```python
from build123d import *

# Parameters (mm, degrees)
SKETCH2_W           = 40
SKETCH2_H           = 20
SKETCH2_R           = 1.5
BOSS_EXTRUDE1_DEPTH = 3
BOSS_EXTRUDE2_DEPTH = 20
SKETCH4_R           = 1.5
CUT_EXTRUDE1_DEPTH  = 20
FILLET2_R           = 2.5


with BuildPart() as part:
    # Sketch2 → Boss-Extrude1 (new body)
    with BuildSketch(Plane(origin=(0, 0, 0), x_dir=(1, 0, 0), z_dir=(0, 1, 0))):
        with Locations((20, 10)):
            Rectangle(SKETCH2_W, SKETCH2_H)
        with Locations(Location((5, 5, 0), (0, 0, 270))):
            Circle(SKETCH2_R, mode=Mode.SUBTRACT)
        with Locations(Location((15, 5, 0), (0, 0, 270))):
            Circle(SKETCH2_R, mode=Mode.SUBTRACT)
        with Locations(Location((15, 15, 0), (0, 0, 270))):
            Circle(SKETCH2_R, mode=Mode.SUBTRACT)
        with Locations(Location((5, 15, 0), (0, 0, 270))):
            Circle(SKETCH2_R, mode=Mode.SUBTRACT)
    extrude(amount=BOSS_EXTRUDE1_DEPTH)

    # Sketch3 → Boss-Extrude2 (add)
    with BuildSketch(Plane(origin=(0, 3, 0), x_dir=(1, 0, 0), z_dir=(0, 1, 0))):
        Polygon((22.097168491, 18), (35.975848148, 4.121320344), (33.854527804, 2), (19.975848148, 15.878679656), align=None)
        Polygon((35.878679656, 8.461129522), (28.461129522, 15.878679656), (30.582449865, 18), (38, 10.582449865), align=None)
    extrude(amount=BOSS_EXTRUDE2_DEPTH)

    # Sketch4 → Cut-Extrude1 (cut)
    with BuildSketch(Plane(origin=(24.291224933, 0, -24.291224933), x_dir=(-0.7071067811865372, 0, -0.7071067811865579), z_dir=(0.7071067811865579, 0, -0.7071067811865372))):
        with Locations((-13.897135624, 18)):
            Circle(SKETCH4_R)
        with Locations((-13.897135624, 13)):
            Circle(SKETCH4_R)
        with Locations((-13.897135624, 8)):
            Circle(SKETCH4_R)
    extrude(amount=-CUT_EXTRUDE1_DEPTH, mode=Mode.SUBTRACT)

    # Fillet2
    fillet2_edges = [part.edges().sort_by_distance(p)[0] for p in [
        (34.915187976, 3, -3.060660172),
        (34.915187976, 23, -3.060660172),
        (36.939339828, 3, -9.521789694),
        (29.521789694, 3, -16.939339828),
        (36.939339828, 23, -9.521789694),
        (29.521789694, 23, -16.939339828),
        (0, 1.5, -20),
        (40, 1.5, 0),
        (0, 1.5, 0),
    ]]
    fillet(fillet2_edges, radius=FILLET2_R)


solid = part.part
```
Check sheet for the modelled part. Datum: model origin and axes. Units: mm. A direction names the side the tool comes from. Round coordinates to 2 decimals unless told otherwise and drop trailing zeros. Order: outer loops, then holes, each group sorted by start corner. A loop starts at its lowest first (then second) coordinate and runs counter-clockwise, first axis right, second up.
1) Section check C-C (z = -15). Give the number of separate pieces and of enclosed holes in the cut face, and give its area (3 significant figures).
2) Go/stop test with flat-tipped pins: pin 1 Ø4 at (x, z) = (15, -15) entering from +Y; pin 2 Ø2.5 at (x, z) = (15, -5) entering from -Y; pin 3 Ø12 at (x, z) = (34.5, -13.5) entering from -Y; pin 4 Ø4 at (x, y) = (25.5, 19) entering from -Z. Record where each tip stops, or that it passes through.
3) Section check B-B (y = 18.5). Record the boundary of the cut face in (x, z), and give its area (3 significant figures).
4) Section check A-A (x = 5). Record the boundary of the cut face in (y, z), and give its area (3 significant figures).
5) Section check D-D (x = 16). Record the boundary of the cut face in (y, z).
6) Tool access check on faces 4 (the flat face through (20, 3, -10)), 5 (the flat face through (21.022, 12.86, -16.924)), 6 (the flat face through (27, 23, -11)), 7 (the flat face through (29.507, 12.895, -16.924)). Record the directions out of +Z, -Z, +X, -X, +Y, -Y that give a thin tool (end or side, any length) a straight path to the whole face; none if there is none.
7) Mould release check, pull along X, two halves, no side actions. Record for faces 1 (the flat face through (26.17, 12.86, -9.684)), 2 (the cylindrical face through (33.914, 12.087, -12.577)), 3 (the cylindrical face through (36.42, 22.25, -10.01)): +X half, -X half, draft (parallel to the pull), parting line (faces both ways), or undercut.
8) Scan lines: line 1 (X direction, y = 0.65, z = -15); line 2 (Y direction, x = 20, z = -14); line 3 (X direction, y = 4.75, z = -11). Record each from-to range of solid material in increasing order.
Result:
1. separate pieces: 3
1. enclosed holes: 0
1. area: 266 mm2
2. pin 1: stops at y = 3
2. pin 2: passes through
2. pin 3: stops at y = 0
2. pin 4: stops at z = -16.6
3. outline: (19.98, -15.88) - (22.1, -18) - (28.88, -11.22) - (26.75, -9.1) - close; (28.46, -15.88) - (30.58, -18) - (33.12, -15.46) - (31, -13.34) - close; (28.75, -7.1) - (30.88, -9.22) - (35.98, -4.12) - (33.85, -2) - close; (33, -11.34) - (35.12, -13.46) - (38, -10.58) - (35.88, -8.46) - close
3. area: 73.4 mm2
4. outline: (0, -20) - (3, -20) - (3, -16.5) - (0, -16.5) - close; (0, -13.5) - (3, -13.5) - (3, -6.5) - (0, -6.5) - close; (0, -3.5) - (3, -3.5) - (3, 0) - (0, 0) - close
4. area: 42.0 mm2
5. outline: (0, -20) - (3, -20) - (3, -16.12) - (0, -16.12) - close; (0, -13.88) - (3, -13.88) - (3, -6.12) - (0, -6.12) - close; (0, -3.88) - (3, -3.88) - (3, 0) - (0, 0) - close
6. face 4: +Y
6. face 5: -Z, -X, +Y
6. face 6: +Z, -Z, +X, -X, +Y
6. face 7: -Z, +Y
7. face 1: -X half
7. face 2: undercut
7. face 3: +X half
8. line 1: x = 0 to 3.5, 6.5 to 13.5, 16.5 to 40
8. line 2: y = 0 to 3
8. line 3: x = 24.85 to 29.1, 33.34 to 37.58
